Source: three-view drawing plus pictorial views. Frame: mm from the lowest corner of the part. Give positions to 0.01 mm unless a question says otherwise; leave off trailing zeros. Loops run counter-clockwise (first coordinate to the right, second up) from the corner with the lowest first, then second, coordinate; pieces in that order, holes last. Notation, with made-up numbers: (0, -20) - (12, -20) arc R27 cw to (12, 11) - close; hole circle Ø6 at (82.25, 46). An arc over 180 degrees is marked (long way). One line per item, written item: value.
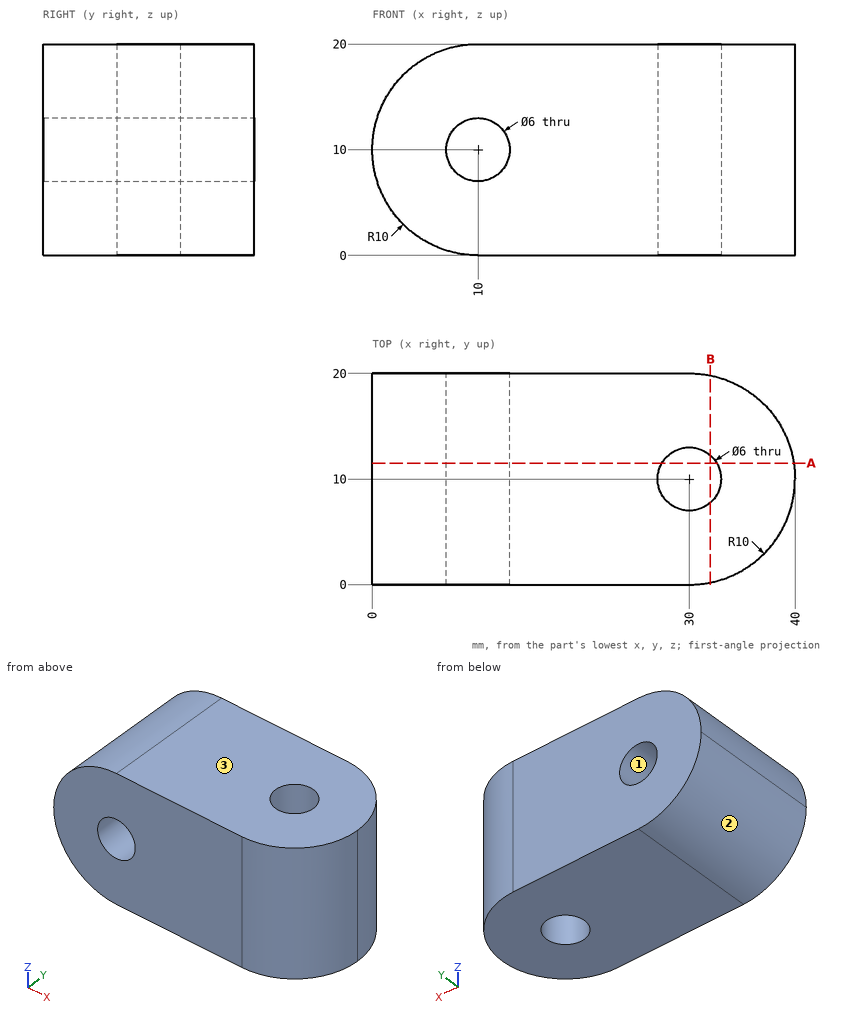
Item 1: Material intervals for L1, parallel to X at y = 11, z = 12.25; L2, parallel to Z at x = 10, y = 13.5, sorted ascending.
Verdict:
L1: x = 0.26 to 8.02, 11.98 to 27.17, 32.83 to 39.95
L2: z = 0 to 7, 13 to 20
Item 2: Draft query along X for the marked faces 1, 2 and 3. Return one class per face: pulls with the +X half, pulls with the -X half, needs draft (parallel to the pull), parting line crosses it, or undercut.
Verdict:
face 1: undercut
face 2: pulls with the -X half
face 3: needs draft
Item 3: Section A-A, the plane y = 11.5. Count the separate pieces of the cut face and the enclosed holes in it, and give its area (3 significant figures).
Verdict:
separate pieces: 2
enclosed holes: 1
area: 623 mm^2
Item 4: Section B-B, the plane x = 32. Output: boundary loops of the cut face in (y, z).
Verdict:
outline: (0.2, 0) - (7.76, 0) - (7.76, 20) - (0.2, 20) - close; (12.24, 0) - (19.8, 0) - (19.8, 20) - (12.24, 20) - close
Item 5: Pin query (flat end, axial travel): P1, Ø4, axis at x = 33.5, z = 15.5, coming from the +Y side; P2, Ø8, axis at y = 15, z = 8, coming from the +X side. Return the tip coordinate at first contact, or that it passes through.
Verdict:
P1: stops at y = 19.89
P2: stops at x = 39.95
